The figure shows three views and two pictorial views of one solid part (mm, origin at its lowest corner). Answer the questions. A direction names the side the tool comes from. Coordinates: 2 decimals unless noted, no trailing zeros. Order: outer loops, then holes, each group sorted by start corner. A loop starts at its lowest first (then second) coordinate and runs counter-clockwise, first axis right, second up. Notation, with made-up numbers: M 11.5,19 L 22.5,19 A18 cw 22.5,39 Z; hole C 82,24.25 d11. An arc over 180 degrees is marked long. Answer in a Markdown table with one row per item. Add a question column.
Item 1: Which of the six approach directions +Z, -Z, +X, -X, +Y, -Y give full straight-line access (tool end or side, diameter ignored) to the marked faces 5 and 6?
Item 2: The mould has two halves that part along X. Classify the marked faces 1, 2, 3 and 4: released by +X, released by -X, zero draft, split by the parting line, or undercut.
Item 3: The part is cut by section D-D (z = 6). Write down the section's boundary in (x, y), then the cut area to 3 significant figures.
Item 4: The part is cut by section C-C (z = 7). Write down the section's boundary in (x, y).
Item 5: Consider line 1 (Y direction, x = 9, z = 2.5); line 2 (Z direction, x = 9, y = 16.3); line 3 (Z direction, x = 9, y = 2.8). Determine where each line is inside the solid, lowest interval first. Write a range as from..to.
Item 6: Flat-ended cylindrical pins translate along their axes: pin 1 Ø1.5 at (x, y) = (10.5, 5.5) entering from +Z; pin 2 Ø3 at (x, z) = (3, 8) entering from +Y; pin 3 Ø1 at (x, z) = (2, 3.5) entering from +Y; pin 4 Ø1.5 at (y, z) = (2, 3) entering from +X. Find the tip coordinate at first contact, or state that the pin passes through.
Item 7: The part is cut by section B-B (x = 9). Write down the section's boundary in (y, z), then the cut area to 3 significant figures.
Item 8: The part is cut by section A-A (y = 9). Write down the section's boundary in (x, z).
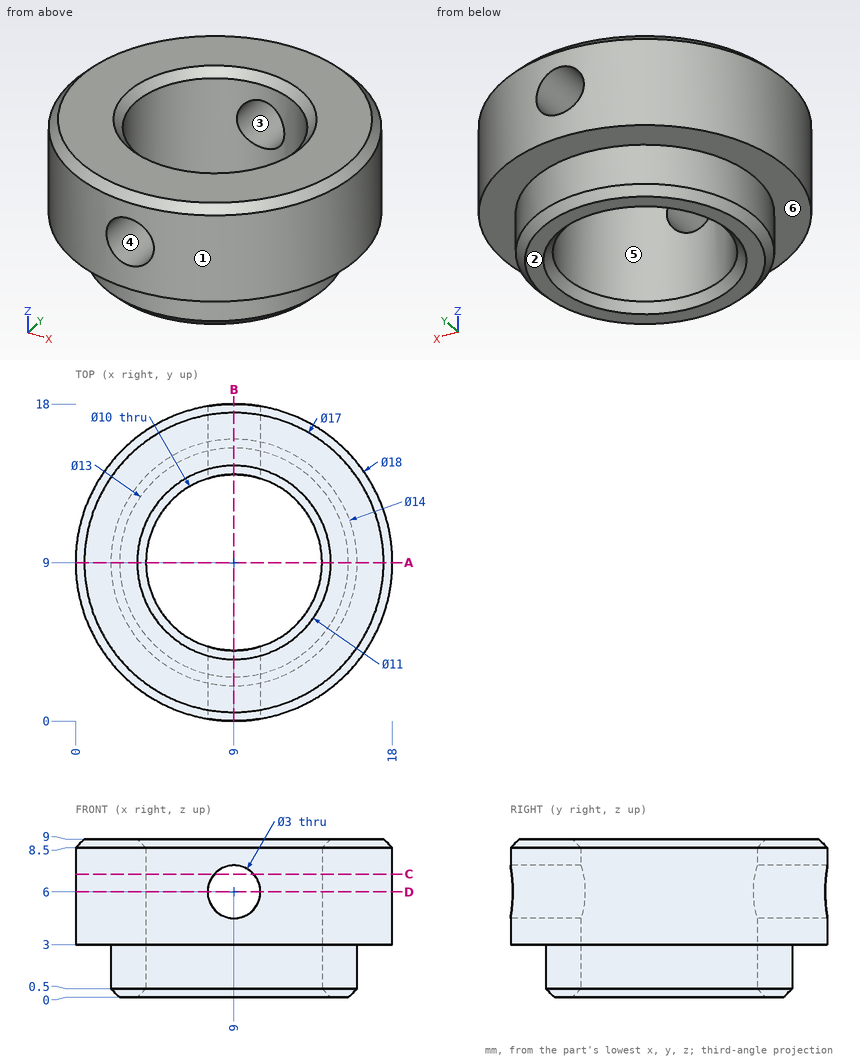
Reply:
| question | item | result |
|---|---|---|
| 1 | face 5 | +Z, -Z |
| 1 | face 6 | -Z |
| 2 | face 1 | split by the parting line |
| 2 | face 2 | zero draft |
| 2 | face 3 | undercut |
| 2 | face 4 | undercut |
| 3 | outline | M 7.5,0.13 L 7.5,4.23 A5 cw 7.5,13.77 L 7.5,17.87 A9 ccw Z; M 10.5,0.13 A9 ccw 10.5,17.87 L 10.5,13.77 A5 cw 10.5,4.23 Z |
| 3 | area | 152 mm2 |
| 4 | outline | M 7.88,0.07 L 7.88,4.13 A5 cw 7.88,13.87 L 7.88,17.93 A9 ccw Z; M 10.12,0.07 A9 ccw 10.12,17.93 L 10.12,13.87 A5 cw 10.12,4.13 Z |
| 5 | line 1 | y = 2..4, 14..16 |
| 5 | line 2 | z = 3..4.5, 7.5..9 |
| 5 | line 3 | z = 0..4.5, 7.5..9 |
| 6 | pin 1 | passes through |
| 6 | pin 2 | stops at y = 16.79 |
| 6 | pin 3 | stops at y = 15.22 |
| 6 | pin 4 | stops at x = 15.48 |
| 7 | outline | M 0,3 L 2,3 L 2,0.5 L 2.5,0 L 3.5,0 L 4,0.5 L 4,4.5 L 0,4.5 Z; M 0,7.5 L 4,7.5 L 4,8.5 L 3.5,9 L 0.5,9 L 0,8.5 Z; M 14,0.5 L 14.5,0 L 15.5,0 L 16,0.5 L 16,3 L 18,3 L 18,4.5 L 14,4.5 Z; M 14,7.5 L 18,7.5 L 18,8.5 L 17.5,9 L 14.5,9 L 14,8.5 Z |
| 7 | area | 35.0 mm2 |
| 8 | outline | M 0,3 L 2,3 L 2,0.5 L 2.5,0 L 3.5,0 L 4,0.5 L 4,8.5 L 3.5,9 L 0.5,9 L 0,8.5 Z; M 14,0.5 L 14.5,0 L 15.5,0 L 16,0.5 L 16,3 L 18,3 L 18,8.5 L 17.5,9 L 14.5,9 L 14,8.5 Z |
